```python
from build123d import *

# Parameters (mm, degrees)
F1_DEPTH = 2.54
F3_DEPTH = 2.54
F5_DEPTH = 1.905


with BuildPart() as f1:
    # F0 (on Right) → F1 (new body, symmetric)
    with BuildSketch(Plane.YZ):
        Polygon((-6.35, 1.020886), (-6.35, 0), (0, 0), (0, 7.62), (-2.54, 7.62), align=None)
    extrude(amount=F1_DEPTH, both=True)

    # F2 (on Right) → F3 (join, symmetric)
    with BuildSketch(Plane.YZ):
        with BuildLine():
            Line((-4.512201, 14.980355), (-2.70435, 8.233363))
            ThreePointArc((-2.70435, 8.233363), (-2.8575, 7.070074), (-1.926637, 7.78435))
            Line((-1.926637, 7.78435), (-1.803965, 7.81722))
            Line((-1.803965, 7.81722), (-1.367615, 9.445697))
            Line((-1.367615, 9.445697), (-2.025016, 11.899149))
            Line((-2.025016, 11.899149), (-3.898838, 15.144705))
            Line((-3.898838, 15.144705), (-4.512201, 14.980355))
        make_face()
    extrude(amount=F3_DEPTH, both=True)

    # F4 (on Right) → F5 (cut, symmetric)
    with BuildSketch(Plane.YZ):
        Polygon((-3.734312, 6.843067), (-6.591812, 1.893732), (-4.932648, 0.935813), (-2.075148, 5.885148), align=None)
    extrude(amount=F5_DEPTH, both=True, mode=Mode.SUBTRACT)


solid = f1.part
```
Model file for the job. Use its own axes, mm. A direction names the side the tool comes from. Round coordinates to 2 decimals unless told otherwise and drop trailing zeros. Write each loop counter-clockwise with the first axis right and the second up, starting at its lowest first coordinate (ties: lowest second). Pieces come first, ordered by that corner, then holes. Notation, with made-up numbers: M -28.75,31.25 L -24.75,31.25 A37 cw -24.75,68.25 Z; hole C 27.5,83.25 d7. An arc over 180 degrees is marked long. Put each result on its own line as item: value.
Item 1: Probe L1, parallel to Z at x = 1, y = -1; L2, parallel to Y at x = 0.2, z = 1.5; L3, parallel to Z at x = -0.4, y = -5.25. List the from-to ranges inside material, lowest first. Write a range as from..to.
Responses:
L1: 0..7.62
L2: -6.07..-5.91, -4.61..0
L3: 0..1.12
Item 2: Flat gauge pins, fed straight in: P1, Ø3, axis at y = -4.5, z = 5, coming from the +X side; P2, Ø1, axis at x = -1, y = -2, coming from the +Z side. Where does each tip first touch, or does it go through?
Responses:
P1: x = 2.54
P2: z = 12.72
Item 3: Tool access for faces 4 (the flat face through (0.04, -3.62, 11.65)), 5 (the flat face through (-2.54, -3, 4)), 6 (the flat face through (0.04, -1.59, 8.62)), 7 (the flat face through (0.03, -2.62, 6.2)), 8 (the flat face through (2.54, -3, 4)): list every direction of +Z, -Z, +X, -X, +Y, -Y with a clear straight run to the whole face (end or side of a thin tool).
Responses:
face 4: +X, -X, -Y
face 5: +Z, -Z, -X, +Y, -Y
face 6: +X, -X, +Y
face 7: -Y
face 8: +Z, -Z, +X, +Y, -Y
Item 4: Cut at A-A (y = -3). List the corners of the cut face in (x, z) (3 decimals).
Responses:
outline: M -2.54,0 L 2.54,0 L 2.54,6.823 L -2.54,6.823 Z; M -2.54,7.182 L 2.54,7.182 L 2.54,8.058 L -2.54,8.058 Z; M -2.54,9.337 L 2.54,9.337 L 2.54,13.588 L -2.54,13.588 Z; hole M -1.905,4.283 L 1.905,4.283 L 1.905,6.419 L -1.905,6.419 Z
Item 5: Cut at D-D (y = -0.75). List the corners of the cut face in (x, z).
Responses:
outline: M -2.54,0 L 2.54,0 L 2.54,7.62 L -2.54,7.62 Z
Item 6: Mould opens along Z. For faces 1 (the flat face through (1.905, -4, 4)), 2 (the flat face through (0.027, -5.49, 1.258)), 3 (the flat face through (0, -6.35, 0.5)) say: +Z half, -Z half, draft (parallel to the pull), parting line (faces both ways), or undercut.
Responses:
face 1: undercut
face 2: +Z half
face 3: draft
Item 7: Cut at C-C (z = 5.5). List the corners of the cut face in (x, y) (3 decimals).
Responses:
outline: M -2.54,-3.764 L -1.905,-3.764 L -1.905,-2.298 L 1.905,-2.298 L 1.905,-3.764 L 2.54,-3.764 L 2.54,0 L -2.54,0 Z
